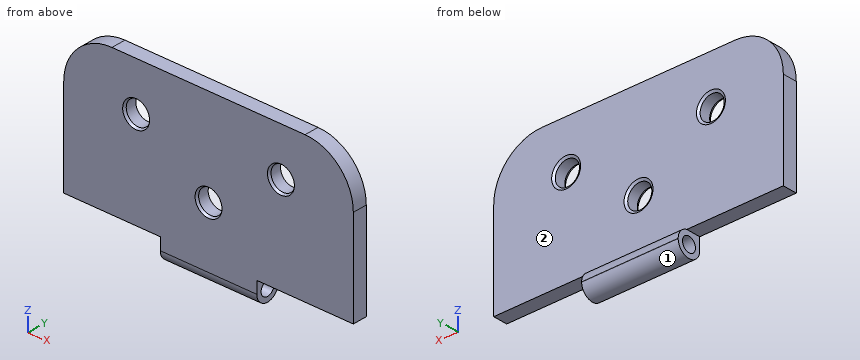
from build123d import *
from OCP.BRepFilletAPI import BRepFilletAPI_MakeChamfer

# Parameters (mm, degrees)
SZKIC1_W                    = 60
SZKIC1_H                    = 30
DODANIE_WYCI_GNI_CIE1_DEPTH = 3
SZKIC2_R                    = 2.5
WYTNIJ_WYCI_GNI_CIE1_DEPTH  = 5
ZAOKR_GLENIE1_R             = 10
SZKIC3_W                    = 20
SZKIC3_H                    = 3
DODANIE_WYCI_GNI_CIE2_DEPTH = 5
SZKIC4_W                    = 20
SZKIC4_H                    = 5
DODANIE_WYCI_GNI_CIE3_DEPTH = 2
ZAOKR_GLENIE2_R             = 2.5
SZKIC5_R                    = 1.5
WYTNIJ_WYCI_GNI_CIE2_DEPTH  = 20
SFAZOWANIE1_SIZE            = 0.5
SFAZOWANIE1_SIZE2           = 0.288675135
SFAZOWANIE2_SIZE            = 0.5
SFAZOWANIE2_SIZE2           = 0.288675135


with BuildPart() as part:
    # Szkic1 → Dodanie-wyciągnięcie1 (new body)
    with BuildSketch(Plane(origin=(0, 0, 0), x_dir=(1, 0, 0), z_dir=(0, 1, 0))):
        Rectangle(SZKIC1_W, SZKIC1_H)
    extrude(amount=DODANIE_WYCI_GNI_CIE1_DEPTH)

    # Szkic2 → Wytnij-wyciągnięcie1 (cut)
    with BuildSketch(Plane(origin=(0, 3, 0), x_dir=(1, 0, 0), z_dir=(0, 1, 0))):
        with Locations(Location((-15, -5, 0), (0, 0, 270))):
            Circle(SZKIC2_R)
        with Locations(Location((15, -5, 0), (0, 0, 270))):
            Circle(SZKIC2_R)
        with Locations(Location((0, 5, 0), (0, 0, 270))):
            Circle(SZKIC2_R)
    extrude(amount=-WYTNIJ_WYCI_GNI_CIE1_DEPTH, mode=Mode.SUBTRACT)

    # Zaokrąglenie1
    zaokr_glenie1_edges = [part.edges().sort_by_distance(p)[0] for p in [
        (30, 1.5, 15),
        (-30, 1.5, 15),
    ]]
    fillet(zaokr_glenie1_edges, radius=ZAOKR_GLENIE1_R)

    # Szkic3 → Dodanie-wyciągnięcie2 (add)
    with BuildSketch(Plane(origin=(0, 0, -15), x_dir=(-1, 0, 0), z_dir=(0, 0, -1))):
        with Locations((0, 1.5)):
            Rectangle(SZKIC3_W, SZKIC3_H)
    extrude(amount=DODANIE_WYCI_GNI_CIE2_DEPTH)

    # Szkic4 → Dodanie-wyciągnięcie3 (add)
    with BuildSketch(Plane(origin=(0, 3, 0), x_dir=(1, 0, 0), z_dir=(0, 1, 0))):
        with Locations((0, 17.5)):
            Rectangle(SZKIC4_W, SZKIC4_H)
    extrude(amount=DODANIE_WYCI_GNI_CIE3_DEPTH)

    # Zaokrąglenie2
    # the kernel refuses this fillet: 2.5 mm, written as the material it takes off along each edge
    with BuildSketch(Plane(origin=(16.25, 0, -20), x_dir=(0, 1, 0), z_dir=(-1, 0, 0)), Plane(origin=(16.25, 5, -20), x_dir=(0, 0, 1), z_dir=(-1, 0, 0))) as zaokr_glenie2_piece_1:
        with BuildLine():
            CenterArc((ZAOKR_GLENIE2_R, -ZAOKR_GLENIE2_R), ZAOKR_GLENIE2_R, 90, 90)
            Line((0, -ZAOKR_GLENIE2_R), (-ZAOKR_GLENIE2_R * 0.02, -ZAOKR_GLENIE2_R))
            Line((-ZAOKR_GLENIE2_R * 0.02, -ZAOKR_GLENIE2_R), (-ZAOKR_GLENIE2_R * 0.02, ZAOKR_GLENIE2_R * 0.02))
            Line((-ZAOKR_GLENIE2_R * 0.02, ZAOKR_GLENIE2_R * 0.02), (ZAOKR_GLENIE2_R, ZAOKR_GLENIE2_R * 0.02))
            Line((ZAOKR_GLENIE2_R, ZAOKR_GLENIE2_R * 0.02), (ZAOKR_GLENIE2_R, 0))
        make_face()
    extrude(amount=32.5, mode=Mode.SUBTRACT)
    with BuildSketch(Plane(origin=(-16.123724357, 5, -15), x_dir=(0, -1.0, -1.666222715356868e-12), z_dir=(1, 0, 0))) as zaokr_glenie2_piece_2:
        with BuildLine():
            CenterArc((2.5, 2.449489743), ZAOKR_GLENIE2_R, 180, 78.463040967)
            Line((0, 2.449489743), (-0.05, 2.449489743))
            Line((-0.05, 2.449489743), (-0.05, 0))
            Line((-0.05, 0), (0, -0.05))
            ThreePointArc((0, -0.05), (1, -0.05), (1.99, -0.048989795))
            Line((1.99, -0.048989795), (2, 0))
        make_face()
    extrude(amount=32.247448714, mode=Mode.SUBTRACT)

    # Szkic5 → Wytnij-wyciągnięcie2 (cut)
    with BuildSketch(Plane(origin=(10, 0, 0), x_dir=(0, 0, -1), z_dir=(1, 0, 0))):
        with Locations((17.474744871, 2.5)):
            Circle(SZKIC5_R)
    extrude(amount=-WYTNIJ_WYCI_GNI_CIE2_DEPTH, mode=Mode.SUBTRACT)

    # Sfazowanie1
    sfazowanie1_edges = [part.edges().sort_by_distance(p)[0] for p in [
        (0, 3, -7.5),
    ]]
    sfazowanie1_side = [part.faces().sort_by_distance(p)[0] for p in [
        (0, 3, -0.380473171),
    ]]
    chamfer(sfazowanie1_edges, length=SFAZOWANIE1_SIZE, length2=SFAZOWANIE1_SIZE2, reference=sfazowanie1_side[0])

    # Sfazowanie2: one chamfer whose edges measure the first distance from different faces: ONE call of the kernel's chamfer builder (chamfer() names one face for all edges)
    sfazowanie2_edges_1 = [part.edges().sort_by_distance(p)[0] for p in [
        (-15, 0, 2.5),
    ]]
    sfazowanie2_side_1 = [part.faces().sort_by_distance(p)[0] for p in [
        (-15, 1.5, 2.5),
    ]]
    sfazowanie2_edges_2 = [part.edges().sort_by_distance(p)[0] for p in [
        (-15, 3, 2.5),
        (15, 3, 2.5),
    ]]
    sfazowanie2_side_2 = [part.faces().sort_by_distance(p)[0] for p in [
        (0, 3, -0.356851383),
    ]]
    sfazowanie2_edges_3 = [part.edges().sort_by_distance(p)[0] for p in [
        (15, 0, 2.5),
    ]]
    sfazowanie2_side_3 = [part.faces().sort_by_distance(p)[0] for p in [
        (15, 1.5, 2.5),
    ]]
    sfazowanie2_edges_4 = [part.edges().sort_by_distance(p)[0] for p in [
        (0, 0, -7.5),
    ]]
    sfazowanie2_side_4 = [part.faces().sort_by_distance(p)[0] for p in [
        (0, 1.355662433, -7.5),
    ]]
    sfazowanie2 = BRepFilletAPI_MakeChamfer(part.part.solid().wrapped)
    for e in sfazowanie2_edges_1:
        sfazowanie2.Add(SFAZOWANIE2_SIZE, SFAZOWANIE2_SIZE2, e.wrapped, sfazowanie2_side_1[0].wrapped)  # the first distance lies on this face
    for e in sfazowanie2_edges_2:
        sfazowanie2.Add(SFAZOWANIE2_SIZE, SFAZOWANIE2_SIZE2, e.wrapped, sfazowanie2_side_2[0].wrapped)  # the first distance lies on this face
    for e in sfazowanie2_edges_3:
        sfazowanie2.Add(SFAZOWANIE2_SIZE, SFAZOWANIE2_SIZE2, e.wrapped, sfazowanie2_side_3[0].wrapped)  # the first distance lies on this face
    for e in sfazowanie2_edges_4:
        sfazowanie2.Add(SFAZOWANIE2_SIZE, SFAZOWANIE2_SIZE2, e.wrapped, sfazowanie2_side_4[0].wrapped)  # the first distance lies on this face
    add(Compound.cast(sfazowanie2.Shape()), mode=Mode.REPLACE)


solid = part.part
Design review of the part built by this model. Coordinates are the model's own, in mm. Face numbers are marked on the shaded views. A direction names the side the tool comes from. Round coordinates to 2 decimals unless told otherwise and drop trailing zeros. Loops run counter-clockwise (first coordinate to the right, second up) from the corner with the lowest first, then second, coordinate; pieces in that order, holes last. Notation, with made-up numbers: (4.5, 42) - (30.5, 42) arc R13 cw to (30.5, 67) - close; hole circle Ø10 at (9.5, 31). An arc over 180 degrees is marked (long way). One line per item, written item: value. Start each with the question number.
1) For the marked faces 1 and 2, list the 3-axis set-ups (+Z, -Z, +X, -X, +Y, -Y) from which the entire face can be reached by the end or side of a thin tool; tool diameter is ignored.
2) Consider section B-B on z = -5. Give the boundary of the cut face in (x, y), then the cut area to 3 significant figures.
3) Insertion check: pin 1 Ø2.5 at (y, z) = (2.5, -17.47) entering from -X; pin 2 Ø3 at (x, y) = (-23.5, 0.5) entering from -Z; pin 3 Ø1.5 at (x, y) = (-7.5, 1) entering from -Z; pin 4 Ø1.5 at (y, z) = (1.5, -18) entering from +X. Each pin has a flat end and moves straight along its axis. Give the tip position at first contact, or say it passes through.
4) To check wall thickness, follow L1, parallel to X at y = 2.9, z = 4; L2, parallel to Y at x = 0.5, z = -17.5; L3, parallel to X at y = 1.85, z = -5. State the ranges of each line that lie inside material, in increasing order. Write a range as from..to.
5) Consider section C-C on x = 0. Give the boundary of the cut face in (y, z), then the cut area to 3 significant figures.
6) Consider section D-D on z = 4. Give the number of separate pieces and of enclosed holes in the cut face, then the cut area to 3 significant figures.
7) Consider section A-A on x = -15. Give the boundary of the cut face in (y, z), then the cut area to 3 significant figures.
Reported:
1. face 1: -Z, +X, -X
1. face 2: +Z, +X, -X, +Y
2. outline: (-30, 0) - (-2.79, 0) - (-2.5, 0.5) - (-2.5, 2.71) - (-3, 3) - (-30, 3) - close; (2.5, 0.5) - (2.79, 0) - (30, 0) - (30, 3) - (3, 3) - (2.5, 2.71) - close
2. area: 165 mm^2
3. pin 1: passes through
3. pin 2: stops at z = -15
3. pin 3: stops at z = -19.88
3. pin 4: stops at x = 10
4. L1: x = -30..-17.64, -12.36..12.36, 17.64..30
4. L2: y = 0..1, 4..5
4. L3: x = -30..-2.5, 2.5..30
5. outline: (0, -17.5) arc R2.5 ccw to (5, -17.5) - (5, -17.45) arc R2.5 ccw to (3, -15) - (3, -8) - (2.71, -7.5) - (0.5, -7.5) - (0, -7.79) - close; (0, -2.21) - (0.5, -2.5) - (2.71, -2.5) - (3, -2) - (3, 15) - (0, 15) - close; hole circle Ø3 at (2.5, -17.47)
5. area: 88.7 mm^2
6. separate pieces: 3
6. enclosed holes: 0
6. area: 152 mm^2
7. outline: (0, -15) - (3, -15) - (3, 2) - (2.71, 2.5) - (0.5, 2.5) - (0, 2.21) - close; (0, 7.79) - (0.5, 7.5) - (2.71, 7.5) - (3, 8) - (3, 15) - (0, 15) - close
7. area: 74.7 mm^2
